Autodesk Inventor part; units mm, degrees
ref_plane "YZ Plane" through (0, 0, 0) normal (1, 0, 0) x (0, 1, 0)
ref_plane "XZ Plane" through (0, 0, 0) normal (0, 1, 0) x (-1, 0, 0)
ref_plane "XY Plane" through (0, 0, 0) normal (0, 0, 1) x (1, 0, 0)
sketch "Sketch4" plane through (0, 0, 0) normal (0, 0, 1) x (1, 0, 0)
  circle A0 centre (0, 0) radius 8
  circle A1 centre (0, 0) radius 10
  line L0 (-10, 0) -> (-10, -14)
  line L1 (10, 0) -> (10, -14)
  line L2 (10, -14) -> (-10, -14)
  line L3 (10, 0) -> (10, 10)
  line L4 (10, 10) -> (0, 10)
  point P0 (10, -7)
  dimension "d12" = 16
  dimension "d13" = 2
  dimension "d14" = 14
  dimension "d17" = 20
extrude "Extrusion3" add sketch "Sketch4" along normal blind 11.25
sketch "Sketch5" plane through (0, 0, 0) normal (0, 0, -1) x (-1, 0, 0)
  circle A0 centre (0, 0) radius 8
  line L0 (0, -19.2142) -> (0, 17.2853)
  arc A1 (10, 0) -> (0, 10) centre (0, 0) ccw
  line L1 (10, 0) -> (10, -14)
  arc A2 (10, 0) -> (0, 10) centre (0, 0) ccw
  line L2 (10, -14) -> (-10, -14)
  circle A3 centre (0, 0) radius 8
  line L3 (-10, 10) -> (0, 10)
  line L4 (-10, -14) -> (-10, 10)
  circle A4 centre (0, 0) radius 7.75
  line L5 (-6, -4.9054) -> (-6, 4.9054)
  line L6 (6, -4.9054) -> (6, 4.9054)
  line L7 (-6, 4.9054) -> (-6, 5.2915)
  line L8 (6, 4.9054) -> (6, 5.2915)
  line L9 (-6, 5.2915) -> (-10, 5.2915)
  line L10 (-10, -14) -> (-10, 10)
  line L11 (6, 5.2915) -> (8.4853, 5.2915)
  point P0 (-10, 0)
  point P1 (-10, 0)
  dimension "d24" = 15.5
  dimension "d25" = 12
extrude "Extrusion4" add sketch "Sketch5" along normal blind 20 contours A0 L0 A4 L8 | A0 L11 A1 L1 L2 L0 | L0 L2 L4 L9 A0 | A0 L7 A4 L0 | A4 L6 | L5 A4 picked at (6.6814, 4.0106) picked at (-6.667, 4.0378)
equation "\"d14\" = DriveMotorHeight - BaseWallThickness"
equation "\"DriveMotorHeight\" = 17"
equation "\"BaseWallThickness\" = 3"
properties part number "MotorMountV1" material "Thermoplastic Resin"
Source: CAD feature listing. Evaluate the final solid. Frame: model axes, mm. A direction names the side the tool comes from. Give positions to 0.01 mm unless a question says otherwise; leave off trailing zeros. Write each loop counter-clockwise with the first axis right and the second up, starting at its lowest first coordinate (ties: lowest second). Pieces come first, ordered by that corner, then holes.
1. Section query B-B (z = 8). Return the cut outline in (x, y).
2. Section query C-C (x = 5.5). Return the cut outline in (y, z), then the cut area to 3 significant figures.
3. Pull-direction query (Y, two-part tool) for faces 1 (the face through (-1.73, 7.81, 5.55)), 2 (the face through (6, 0, -10)), 3 (the face through (0, -14, -5)); classes: +Y half, -Y half, draft (parallel to the pull), parting line (faces both ways), or undercut.
4. Section query A-A (y = 6.75). Return the cut outline in (x, z).
5. Section query D-D (y = -2). Return the cut outline in (x, z).
6. Access query for faces 4 (the face through (8, 5.292, -10)), 5 (the face through (-9.109, 4.126, -1.122)), 6 (the face through (-6.5, -0.8, 0)), 7 (the face through (-6, 0, -10)). Directions: +Z, -Z, +X, -X, +Y, -Y. A direction counts if a zero-diameter tool reaches every point of the face in a straight line with its end or side. Return the directions, or none.
7. Material intervals for line 1 along X through (y, z) = (0, 6.25); line 2 along Y through (x, z) = (-0.25, 8.5); line 3 along X through (y, z) = (-3, -9), sorted ascending.
8. First-contact query: pin 1 (1.5 mm diameter, centred on x = -7, y = 7, fed in from -Z); pin 2 (6.5 mm diameter, centred on x = 4, y = 0, fed in from +Z); pin 3 (1.2 mm diameter, centred on x = -7.5, z = -7, fed in from +Y). Flat tips, straight axial feed; report the tip coordinate or a pass-through.
Output values:
1. outline: (-10, -14) - (10, -14) - (10, 10) - (0, 10) arc R10 ccw to (-10, 0) - close; hole circle Ø16 at (0, 0)
2. outline: (-14, -20) - (-5.46, -20) - (-5.46, 0) - (-5.81, 0) - (-5.81, 11.25) - (-14, 11.25) - close; (5.81, 0) - (10, 0) - (10, 11.25) - (5.81, 11.25) - close
2. area: 310 mm2
3. face 1: undercut
3. face 2: draft
3. face 3: -Y half
4. outline: (-7.38, 0) - (-4.29, 0) - (-4.29, 11.25) - (-7.38, 11.25) - close; (4.29, 0) - (10, 0) - (10, 11.25) - (4.29, 11.25) - close
5. outline: (-10, -20) - (-6, -20) - (-6, 0) - (-7.75, 0) - (-7.75, 11.25) - (-10, 11.25) - close; (6, -20) - (10, -20) - (10, 11.25) - (7.75, 11.25) - (7.75, 0) - (6, 0) - close
6. face 4: -Z, +X, -X, +Y
6. face 5: +Z, -Z, -X, +Y
6. face 6: +Z
6. face 7: +Z, -Z, +Y
7. line 1: x = -10 to -8, 8 to 10
7. line 2: y = -14 to -8, 8 to 10
7. line 3: x = -10 to -6, 6 to 10
8. pin 1: stops at z = 0
8. pin 2: stops at z = 0
8. pin 3: stops at y = 5.29
